Geometry check sheet. Reference: the model listing, model coordinates, mm. A direction names the side the tool comes from. Round coordinates to 2 decimals unless told otherwise and drop trailing zeros. Write each loop counter-clockwise with the first axis right and the second up, starting at its lowest first coordinate (ties: lowest second). Pieces come first, ordered by that corner, then holes. Notation, with made-up numbers: M 66.5,48 L 79.5,48 A28 ccw 79.5,74 Z; hole C -25.5,-2.5 d3. An arc over 180 degrees is marked long. Use a Markdown table: item, result.
```python
from build123d import *

# Parameters (mm, degrees)
BOX007_W          = 10
BOX007_H          = 12
BOX007_DEPTH      = 10
CYLINDER003_R     = 6
CYLINDER003_DEPTH = 10
CYLINDER002_R     = 6
CYLINDER002_DEPTH = 10
BOX006_W          = 10
BOX006_H          = 12
BOX006_DEPTH      = 10
CYLINDER_R        = 6
CYLINDER_DEPTH    = 10
CYLINDER001_R     = 6
CYLINDER001_DEPTH = 10
EXTRUDE002_DEPTH  = 20
EXTRUDE003_DEPTH  = 20
EXTRUDE004_DEPTH  = 20
EXTRUDE005_DEPTH  = 20
EXTRUDE006_DEPTH  = 20
EXTRUDE001_DEPTH  = 20
EXTRUDE_DEPTH     = 20
BOX_W             = 44
BOX_H             = 90
BOX_DEPTH         = 2


with BuildPart() as cube007:
    # Box007 → Box007 (new body)
    with BuildSketch(Plane(origin=(17, 13.5, 0), x_dir=(1, 0, 0), z_dir=(0, 0, 1))):
        with Locations((5, 6)):
            Rectangle(BOX007_W, BOX007_H)
    extrude(amount=BOX007_DEPTH)


with BuildPart() as fusion003:
    # Cylinder003 → Cylinder003 (new body)
    with BuildSketch(Plane(origin=(18, 19.5, 0), x_dir=(1, 0, 0), z_dir=(0, 0, 1))):
        Circle(CYLINDER003_R)
    extrude(amount=CYLINDER003_DEPTH)

    # Fusion003: union Cube007
    add(cube007.part)


with BuildPart() as fusion002:
    # Cylinder002 → Cylinder002 (new body)
    with BuildSketch(Plane(origin=(26, 19.5, 0), x_dir=(1, 0, 0), z_dir=(0, 0, 1))):
        Circle(CYLINDER002_R)
    extrude(amount=CYLINDER002_DEPTH)

    # Fusion002: union Fusion003
    add(fusion003.part)


with BuildPart() as fusion002_1:
    # Fusion002 placement: moved
    add(fusion002.part.moved(Location((0, 27, 0))))


with BuildPart() as cube006:
    # Box006 → Box006 (new body)
    with BuildSketch(Plane(origin=(17, 13.5, 0), x_dir=(1, 0, 0), z_dir=(0, 0, 1))):
        with Locations((5, 6)):
            Rectangle(BOX006_W, BOX006_H)
    extrude(amount=BOX006_DEPTH)


with BuildPart() as fusion:
    # Cylinder → Cylinder (new body)
    with BuildSketch(Plane(origin=(18, 19.5, 0), x_dir=(1, 0, 0), z_dir=(0, 0, 1))):
        Circle(CYLINDER_R)
    extrude(amount=CYLINDER_DEPTH)

    # Fusion: union Cube006
    add(cube006.part)


with BuildPart() as fusion001:
    # Cylinder001 → Cylinder001 (new body)
    with BuildSketch(Plane(origin=(26, 19.5, 0), x_dir=(1, 0, 0), z_dir=(0, 0, 1))):
        Circle(CYLINDER001_R)
    extrude(amount=CYLINDER001_DEPTH)

    # Fusion001: union Fusion
    add(fusion.part)


with BuildPart() as extrude_c:
    # Sketch007 (on Face6 of Box005) → Extrude002 (new body)
    with BuildSketch(Plane.XY.offset(10)):
        Polygon((38, 30), (42, 26), (42, 13), (38, 9), (34, 13), (34, 26), align=None)
    extrude(amount=EXTRUDE002_DEPTH)


with BuildPart() as extrude_c_1:
    # Extrude002 placement: moved
    add(extrude_c.part.moved(Location((0, 0, -18))))


with BuildPart() as extrude_d:
    # Sketch004 (on Face6 of Box002) → Extrude003 (new body)
    with BuildSketch(Plane.XY.offset(10)):
        Polygon((10, 11), (6, 7), (10, 3), (34, 3), (38, 7), (34, 11), align=None)
    extrude(amount=EXTRUDE003_DEPTH)


with BuildPart() as extrude_d_1:
    # Extrude003 placement: moved
    add(extrude_d.part.moved(Location((0, 0, -20))))


with BuildPart() as extrude_e:
    # Sketch005 (on Face6 of Box003) → Extrude004 (new body)
    with BuildSketch(Plane.XY.offset(10)):
        Polygon((6, 30), (10, 26), (10, 13), (6, 9), (2, 13), (2, 26), align=None)
    extrude(amount=EXTRUDE004_DEPTH)


with BuildPart() as extrude_e_1:
    # Extrude004 placement: moved
    add(extrude_e.part.moved(Location((0, 0, -20))))


with BuildPart() as extrude_f:
    # Sketch (on Face6 of Box) → Extrude005 (new body)
    with BuildSketch(Plane.XY.offset(2)):
        Polygon((6, 81), (10, 77), (10, 64), (6, 60), (2, 64), (2, 77), align=None)
    extrude(amount=EXTRUDE005_DEPTH)


with BuildPart() as extrude_f_1:
    # Extrude005 placement: moved
    add(extrude_f.part.moved(Location((0, 0, -12))))


with BuildPart() as extrude_g:
    # Sketch002 (on Face6 of Box) → Extrude006 (new body)
    with BuildSketch(Plane.XY.offset(2)):
        Polygon((10, 61), (6, 57), (10, 53), (34, 53), (38, 57), (34, 61), align=None)
    extrude(amount=EXTRUDE006_DEPTH)


with BuildPart() as extrude_g_1:
    # Extrude006 placement: moved
    add(extrude_g.part.moved(Location((0, 0, -13))))


with BuildPart() as extrude_b:
    # Sketch006 (on Face6 of Box004) → Extrude001 (new body)
    with BuildSketch(Plane.XY.offset(10)):
        Polygon((38, 58), (42, 54), (42, 30), (38, 26), (34, 30), (34, 54), align=None)
    extrude(amount=EXTRUDE001_DEPTH)


with BuildPart() as extrude_b_1:
    # Extrude001 placement: moved
    add(extrude_b.part.moved(Location((0, 0, -17))))


with BuildPart() as extrude_a:
    # Sketch003 (on Face6 of Box001) → Extrude (new body)
    with BuildSketch(Plane.XY.offset(10)):
        Polygon((10, 63), (6, 59), (10, 55), (34, 55), (38, 59), (34, 63), align=None)
    extrude(amount=EXTRUDE_DEPTH)


with BuildPart() as extrude_a_1:
    # Extrude placement: moved
    add(extrude_a.part.moved(Location((0, 0, -14))))


with BuildPart() as obj1:
    # Box → Box (new body)
    with BuildSketch(Plane.XY):
        with Locations((22, 45)):
            Rectangle(BOX_W, BOX_H)
    extrude(amount=BOX_DEPTH)

    # Cut: cut Extrude_A
    add(extrude_a_1.part, mode=Mode.SUBTRACT)

    # Cut001: cut Extrude_B
    add(extrude_b_1.part, mode=Mode.SUBTRACT)

    # Cut002: cut Extrude_G
    add(extrude_g_1.part, mode=Mode.SUBTRACT)

    # Cut003: cut Extrude_F
    add(extrude_f_1.part, mode=Mode.SUBTRACT)

    # Cut004: cut Extrude_E
    add(extrude_e_1.part, mode=Mode.SUBTRACT)

    # Cut005: cut Extrude_D
    add(extrude_d_1.part, mode=Mode.SUBTRACT)

    # Cut006: cut Extrude_C
    add(extrude_c_1.part, mode=Mode.SUBTRACT)

    # Cut007: cut Fusion001
    add(fusion001.part, mode=Mode.SUBTRACT)

    # Cut008: cut Fusion002
    add(fusion002_1.part, mode=Mode.SUBTRACT)


solid = obj1.part
```
Item 1: Mould release check, pull along X, two halves, no side actions. Record for faces 3 (the face through (22, 0, 1)), 4 (the face through (22, 52.5, 1)), 5 (the face through (42, 20, 1)): +X half, -X half, draft (parallel to the pull), parting line (faces both ways), or undercut.
Outcome:
| item | result |
|---|---|
| face 3 | draft |
| face 4 | undercut |
| face 5 | undercut |
Item 2: Cross-section at A-A, the plane y = 75. Record the cut outline in (x, z), and give its area (3 significant figures).
Outcome:
| item | result |
|---|---|
| outline | M 0,0 L 2,0 L 2,2 L 0,2 Z; M 10,0 L 44,0 L 44,2 L 10,2 Z |
| area | 72.0 mm2 |
Item 3: Cross-section at C-C, the plane x = 19. Record the cut outline in (y, z).
Outcome:
| item | result |
|---|---|
| outline | M 0,0 L 3,0 L 3,2 L 0,2 Z; M 11,0 L 13.5,0 L 13.5,2 L 11,2 Z; M 25.5,0 L 40.5,0 L 40.5,2 L 25.5,2 Z; M 52.5,0 L 53,0 L 53,2 L 52.5,2 Z; M 63,0 L 90,0 L 90,2 L 63,2 Z |
Item 4: Cross-section at D-D, the plane y = 22.5. Record the cut outline in (x, z).
Outcome:
| item | result |
|---|---|
| outline | M 0,0 L 2,0 L 2,2 L 0,2 Z; M 10,0 L 12.8,0 L 12.8,2 L 10,2 Z; M 31.2,0 L 34,0 L 34,2 L 31.2,2 Z; M 42,0 L 44,0 L 44,2 L 42,2 Z |
Item 5: Cross-section at B-B, the plane x = 41. Record the cut outline in (y, z).
Outcome:
| item | result |
|---|---|
| outline | M 0,0 L 12,0 L 12,2 L 0,2 Z; M 27,0 L 29,0 L 29,2 L 27,2 Z; M 55,0 L 90,0 L 90,2 L 55,2 Z |
Item 6: Access from +Z, -Z, +X, -X, +Y, -Y to the whole of each face (thin tool, end or side, straight path). Record for faces 1 (the face through (22, 66, 0)), 2 (the face through (32, 19.4, 1)).
Outcome:
| item | result |
|---|---|
| face 1 | -Z, +X, -X, +Y, -Y |
| face 2 | +Z, -Z |
Item 7: Material ranges on line 1 along Y through (x, z) = (11.5, 1); line 2 along Y through (x, z) = (17.5, 1.65); line 3 along X through (y, z) = (36.5, 1.1), recorded low to high. Write a range as from..to.
Outcome:
| item | result |
|---|---|
| line 1 | y = 0..3, 11..53, 63..90 |
| line 2 | y = 0..3, 11..13.5, 25.5..40.5, 52.5..53, 63..90 |
| line 3 | x = 0..34, 42..44 |
